Part model, mm, in its own coordinate system. Face numbers are marked on the shaded views. A direction names the side the tool comes from. Give positions to 0.01 mm unless a question says otherwise; leave off trailing zeros. Loops run counter-clockwise (first coordinate to the right, second up) from the corner with the lowest first, then second, coordinate; pieces in that order, holes last. Notation, with made-up numbers: (-9.5, -16) -> (41.5, -16) arc R16 ccw to (41.5, -7) -> close; hole circle Ø2 at (-15.75, 82). An arc over 180 degrees is marked (long way). One line per question, with ' | ' between items.
Autodesk Inventor part; units mm, degrees
ref_plane "YZ Plane" through (0, 0, 0) normal (1, 0, 0) x (0, 1, 0)
ref_plane "XZ Plane" through (0, 0, 0) normal (0, 1, 0) x (-1, 0, 0)
ref_plane "XY Plane" through (0, 0, 0) normal (0, 0, 1) x (1, 0, 0)
sketch "Boceto1" plane through (0, 0, 0) normal (0, 0, 1) x (1, 0, 0)
  line L0 (0, 0) -> (0, 40.1) construction
  line L1 (7.5, 0) -> (7.5, 40.1)
  line L2 (-7.5, 40.1) -> (-7.5, 0)
  arc A0 (-7.5, 0) -> (7.5, 0) centre (0, 0) ccw
  arc A1 (7.5, 40.1) -> (-7.5, 40.1) centre (0, 40.1) ccw
  point P0 (0, 20.05)
  dimension "d0" = 40.1
  dimension "d1" = 15
extrude "Extrusión1" add sketch "Boceto1" along normal blind 18
sketch "Boceto2" plane through (0, 0, 0) normal (0, 0, -1) x (-1, 0, 0)
  arc A0 (7.5, 40.1) -> (-7.5, 40.1) centre (0, 40.1) ccw
  line L0 (0, 40.1) -> (0, 24.6)
  line L1 (0, 24.6) -> (-3.5, 24.6)
  line L2 (-3.5, 24.6) -> (3.5, 24.6)
  line L3 (3.5, 24.6) -> (3.5, 40.1)
  line L4 (3.5, 40.1) -> (-3.5, 40.1)
  line L5 (-3.5, 40.1) -> (-3.5, 24.6)
  point P0 (0, 0)
  dimension "d4" = 15.5
  dimension "d5" = 3.5
  dimension "d6" = 7
extrude "Extrusión2" cut sketch "Boceto2" against normal blind 17
sketch "Boceto3" plane through (0, 0, 0) normal (0, 0, -1) x (-1, 0, 0)
  line L0 (-3.5, 40.1) -> (3.5, 40.1)
  line L1 (0, 40.1) -> (0, 41.1)
  line L2 (7.5, 40.1) -> (7.5, 0)
  line L3 (7.5, 20.05) -> (-7.5, 20.05)
  line L4 (-7.5, 0) -> (-7.5, 40.1)
  line L5 (0, 0) -> (0, -1)
  line L6 (-5.3571, 42.7751) -> (-5.3571, 44.0501)
  line L7 (-5.3571, -2.6751) -> (-5.3571, -3.9501)
  line L8 (-5.3571, 44.0501) -> (-5.3571, 45.3489)
  arc A0 (7.5, 40.1) -> (-7.5, 40.1) centre (0, 40.1) ccw
  arc A1 (5.3571, 45.3489) -> (-5.3571, 45.3489) centre (0, 40.1) ccw
  arc A2 (-5.3571, -5.2489) -> (5.3571, -5.2489) centre (0, 0) ccw
  line L9 (-5.3571, -3.9501) -> (-5.3571, -5.2489)
  line L10 (5.3571, -4.6499) -> (5.3571, -5.2489)
  arc A3 (-7.5, 0) -> (7.5, 0) centre (0, 0) ccw
  line L11 (5.3571, 45.3489) -> (5.3571, 42.7751)
  line L12 (-5.3571, 42.7751) -> (5.3571, 42.7751)
  line L13 (5.3571, -4.6499) -> (5.3571, -2.6751)
  line L14 (-5.3571, -2.6751) -> (5.3571, -2.6751)
  point P0 (4.6429, 42.4001)
  dimension "d10" = 1
extrude "Extrusión3" add sketch "Boceto3" along normal blind 8 contours L11 L12 L6 L8 A0 | A2 L9 L7 L14 L13 L10
sketch "Boceto4" plane through (0, 0, 0) normal (0, 0, -1) x (-1, 0, 0)
  line L0 (2.5, 24.6) -> (2.5, -1)
  line L1 (2.5, -1) -> (-2.5, -1)
  line L2 (-2.5, -1) -> (-2.5, 24.6)
  line L3 (-2.5, 24.6) -> (2.5, 24.6)
  line L4 (3.5, 24.6) -> (-3.5, 24.6)
  point P0 (0, 0)
extrude "Extrusión4" cut sketch "Boceto4" against normal blind 5
fillet "Empalme1" radius 1 4 edges at (0, 47.6, 18) (-7.5, 20.05, 18) (0, -7.5, 18) (7.5, 20.05, 18)
properties part number "Tapa carcasa Luis"
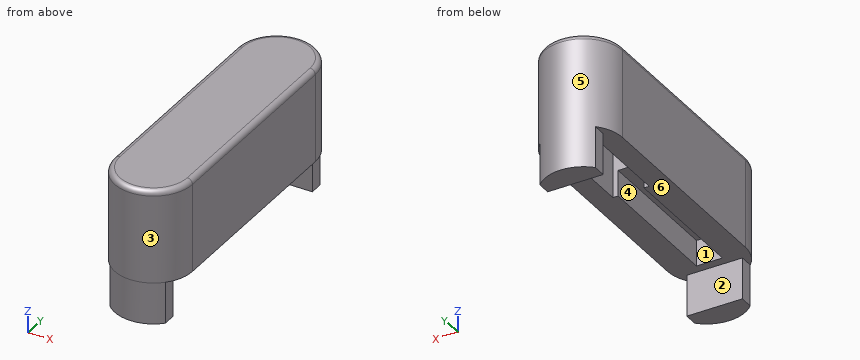
1) Pin check, flat tips, straight feed: P1, Ø2, axis at x = 4, z = 14, coming from the -Y side; P2, Ø2, axis at x = 0, y = 36, coming from the -Z side; P3, Ø2, axis at x = 3.5, z = 8, coming from the -Y side. Stop position of each tip, or through.
Found:
P1: y = -6.87 | P2: z = 17 | P3: y = -7.07
2) Tool access for the marked faces 1, 2 and 3: list every direction of +Z, -Z, +X, -X, +Y, -Y with a clear straight run to the whole face (end or side of a thin tool).
Found:
face 1: -Z | face 2: -Z, +X, -X | face 3: +Z, -Z, -Y
3) Saw through at A-A (z = -3.5). Give the cut face in (x, y), and give its area (3 significant figures).
Found:
outline: (-5.36, -5.25) arc R7.5 ccw to (5.36, -5.25) -> (5.36, -2.68) -> (-5.36, -2.68) -> close; (-5.36, 42.78) -> (5.36, 42.78) -> (5.36, 45.35) arc R7.5 ccw to (-5.36, 45.35) -> close | area: 88.4 mm2
4) Pull direction X, two halves, no side cores. Call the marked faces 4, 5 and 6: pulls with the +X half, pulls with the -X half, needs draft (parallel to the pull), parting line crosses it, or undercut.
Found:
face 4: undercut | face 5: parting line crosses it | face 6: needs draft
5) Saw through at D-D (z = 7.75). Give the cut face in (x, y), and give its area (3 significant figures).
Found:
outline: (-7.5, 0) arc R7.5 ccw to (7.5, 0) -> (7.5, 40.1) arc R7.5 ccw to (-7.5, 40.1) -> close; hole (-3.5, 24.6) -> (3.5, 24.6) -> (3.5, 40.1) -> (-3.5, 40.1) -> close | area: 670 mm2
6) Saw through at B-B (x = 0). Give the cut face in (y, z), and give its area (3 significant figures).
Found:
outline: (-7.5, -8) -> (-2.68, -8) -> (-2.68, 0) -> (-1, 0) -> (-1, 5) -> (24.6, 5) -> (24.6, 17) -> (40.1, 17) -> (40.1, 0) -> (42.78, 0) -> (42.78, -8) -> (47.6, -8) -> (47.6, 17) arc R1 ccw to (46.6, 18) -> (-6.5, 18) arc R1 ccw to (-7.5, 17) -> close | area: 677 mm2
7) Saw through at C-C (y = 21.5). Give the cut face in (x, z).
Found:
outline: (-7.5, 0) -> (-2.5, 0) -> (-2.5, 5) -> (2.5, 5) -> (2.5, 0) -> (7.5, 0) -> (7.5, 17) arc R1 ccw to (6.5, 18) -> (-6.5, 18) arc R1 ccw to (-7.5, 17) -> close
8) Drill centre lines: line 1 (X direction, y = 24, z = 1.75); line 2 (X direction, y = 25, z = 9.25); line 3 (Y direction, x = 0.25, z = 16.25). Where is each one in solid material? Low to high.
Found:
line 1: -7.5 to -2.5, 2.5 to 7.5 | line 2: -7.5 to -3.5, 3.5 to 7.5 | line 3: -7.5 to 24.6, 40.1 to 47.6
